Design review of the part built by this model. Coordinates are the model's own, in mm. Face numbers are marked on the shaded views. A direction names the side the tool comes from. Round coordinates to 2 decimals unless told otherwise and drop trailing zeros. Loops run counter-clockwise (first coordinate to the right, second up) from the corner with the lowest first, then second, coordinate; pieces in that order, holes last. Notation, with made-up numbers: (-10.5, 50) - (29.5, 50) arc R29 cw to (29.5, 84) - close; hole circle Ø9 at (-20, 31.5). An arc over 180 degrees is marked (long way). Return JSON: item names as keys, results as strings. Group by question number.
(1) We need section C-C, the plane z = -1.75. Write out the cut boundary in (x, y), and give its area (3 significant figures).
(2) Wall thickness on L1, parallel to X at y = 7.5, z = 10.15; L2, parallel to X at y = 10, z = 12; L3, parallel to Y at x = 78.5, z = 1: over which ranges is each line inside the solid? List them lowest first. Write a range as [from, to].
(3) For the marked faces 1 and 2, list the 3-axis set-ups (+Z, -Z, +X, -X, +Y, -Y) from which the entire face can be reached by the end or side of a thin tool; tool diameter is ignored.
(4) We need section B-B, the plane y = 22. Write out the cut boundary in (x, z).
(5) The part is to be moulded in two halves that separate along X. For the marked faces 3, 4, 5 and 6, say which applies: pulls with the +X half, pulls with the -X half, needs draft (parallel to the pull), parting line crosses it, or undercut.
(6) We need section D-D, the plane y = 51.5. Write out the cut boundary in (x, z), and give its area (3 significant figures).
(7) We need section A-A, the plane z = 2.25. Write out the cut boundary in (x, y).
(8) Clearance check with flat-ended pins moving along their axes: pin 1 (1 mm diameter, centred on x = 110.5, y = 28, fed in from -Z); pin 2 (5 mm diameter, centred on x = 87.5, y = 38.99, fed in from -Z); pin 3 (3 mm diameter, centred on x = 86.5, z = -2.5, fed in from -Y). State where each tip first meets the part, or that it passes through.
from build123d import *

# Parameters (mm, degrees)
SKETCH1_W           = 80
SKETCH1_H           = 18
SKETCH1_R           = 3
BOSS_EXTRUDE1_DEPTH = 20
SKETCH1_3_W         = 27.5
SKETCH1_3_H         = 18
SKETCH1_3_W_2       = 25
SKETCH1_3_R         = 3.5
BOSS_EXTRUDE2_DEPTH = 47
BOSS_EXTRUDE3_START = 47
SKETCH1_6_W         = 80
SKETCH1_6_H         = 18
BOSS_EXTRUDE3_DEPTH = 10
SKETCH2_R           = 5.5
SKETCH2_R_2         = 4.475
SKETCH2_R_3         = 3
BOSS_EXTRUDE4_DEPTH = 25
SKETCH2_6_R         = 10.5
SKETCH2_6_R_2       = 3
CUT_EXTRUDE5_DEPTH  = 161.097543738
SKETCH1_8_R         = 3
CUT_EXTRUDE6_DEPTH  = 57
CUT_EXTRUDE13_START = 27
SKETCH1_12_R        = 3
CUT_EXTRUDE13_DEPTH = 30
CUT_EXTRUDE14_START = -18
SKETCH2_7_W         = 9.3
SKETCH2_7_H         = 5
CUT_EXTRUDE14_DEPTH = 10


with BuildPart() as part:
    # Sketch1 → Boss-Extrude1 (new body)
    with BuildSketch(Plane(origin=(0, 0, 0), x_dir=(1, 0, 0), z_dir=(0, 1, 0))):
        with Locations((107.5033, -9)):
            Rectangle(SKETCH1_W, SKETCH1_H)
        with Locations(Location((135.5033, -10.15, 0), (0, 0, 270))):
            Circle(SKETCH1_R, mode=Mode.SUBTRACT)
        with Locations(Location((79.5033, -10.15, 0), (0, 0, 270))):
            Circle(SKETCH1_R, mode=Mode.SUBTRACT)
    extrude(amount=BOSS_EXTRUDE1_DEPTH)

    # Sketch1<3> → Boss-Extrude2 (add)
    # profile 1 of 11: a face of its own
    with BuildSketch(Plane(origin=(0, 0, 0), x_dir=(1, 0, 0), z_dir=(0, 1, 0))):
        with Locations((133.7533, -9)):
            Rectangle(SKETCH1_3_W, SKETCH1_3_H)
        Polygon((133.136163896, -6.05), (137.870436104, -6.05), (140.237572207, -10.15), (137.870436104, -14.25), (133.136163896, -14.25), (130.769027793, -10.15), align=None, mode=Mode.SUBTRACT)
    # profile 2 of 11: a face of its own
    with BuildSketch(Plane(origin=(0, 0, 0), x_dir=(1, 0, 0), z_dir=(0, 1, 0))):
        with Locations((81.2533, -9)):
            Rectangle(SKETCH1_3_W, SKETCH1_3_H)
        Polygon((81.88895579, -14.295097543), (77.154690915, -14.303429856), (74.780342483, -10.207602362), (77.140258926, -6.103442556), (81.874523801, -6.095110243), (84.248872233, -10.190937737), align=None, mode=Mode.SUBTRACT)
    # profile 3 of 11: a face of its own
    with BuildSketch(Plane(origin=(0, 0, 0), x_dir=(1, 0, 0), z_dir=(0, 1, 0))):
        with Locations((107.5033, -9)):
            Rectangle(SKETCH1_3_W_2, SKETCH1_3_H)
        with BuildLine():
            ThreePointArc((111.0033, -10.75), (107.5033, -14.25), (104.0033, -10.75))
            Line((104.0033, -10.75), (104.0033, -7.25))
            ThreePointArc((104.0033, -7.25), (107.5033, -3.75), (111.0033, -7.25))
            Line((111.0033, -7.25), (111.0033, -10.75))
        make_face(mode=Mode.SUBTRACT)
    # profile 4 of 11: a face of its own
    with BuildSketch(Plane(origin=(0, 0, 0), x_dir=(1, 0, 0), z_dir=(0, 1, 0))):
        with Locations((107.5033, -10.75)):
            Circle(SKETCH1_3_R)
    # profile 5 of 11: a face of its own
    with BuildSketch(Plane(origin=(0, 0, 0), x_dir=(1, 0, 0), z_dir=(0, 1, 0))):
        with Locations((107.5033, -7.25)):
            Circle(SKETCH1_3_R)
    # profile 6 of 11: a face of its own
    with BuildSketch(Plane(origin=(0, 0, 0), x_dir=(1, 0, 0), z_dir=(0, 1, 0))):
        with Locations((107.5033, -7.25)):
            Circle(SKETCH1_3_R)
    # profile 7 of 11: a face of its own
    with BuildSketch(Plane(origin=(0, 0, 0), x_dir=(1, 0, 0), z_dir=(0, 1, 0))):
        with Locations((107.5033, -10.75)):
            Circle(SKETCH1_3_R)
    # profile 8 of 11: a face of its own
    with BuildSketch(Plane(origin=(0, 0, 0), x_dir=(1, 0, 0), z_dir=(0, 1, 0))):
        with BuildLine():
            Line((104.0033, -7.25), (104.0033, -10.75))
            ThreePointArc((104.0033, -10.75), (104.122559608, -9.844133342), (104.472211087, -9))
            ThreePointArc((104.472211087, -9), (104.122559608, -8.155866658), (104.0033, -7.25))
        make_face()
    # profile 9 of 11: a face of its own
    with BuildSketch(Plane(origin=(0, 0, 0), x_dir=(1, 0, 0), z_dir=(0, 1, 0))):
        with BuildLine():
            ThreePointArc((110.534388913, -9), (110.884040392, -9.844133342), (111.0033, -10.75))
            Line((111.0033, -10.75), (111.0033, -7.25))
            ThreePointArc((111.0033, -7.25), (110.884040392, -8.155866658), (110.534388913, -9))
        make_face()
    # profile 10 of 11: a face of its own
    with BuildSketch(Plane(origin=(0, 0, 0), x_dir=(1, 0, 0), z_dir=(0, 1, 0))):
        with Locations((107.5033, -10.75)):
            Circle(SKETCH1_3_R)
    # profile 11 of 11: a face of its own
    with BuildSketch(Plane(origin=(0, 0, 0), x_dir=(1, 0, 0), z_dir=(0, 1, 0))):
        with Locations((107.5033, -7.25)):
            Circle(SKETCH1_3_R)
    extrude(amount=BOSS_EXTRUDE2_DEPTH)

    # Sketch1<6> → Boss-Extrude3 (add)
    with BuildSketch(Plane(origin=(0, 0, 0), x_dir=(1, 0, 0), z_dir=(0, 1, 0)).offset(BOSS_EXTRUDE3_START)):
        with Locations((107.5033, -9)):
            Rectangle(SKETCH1_6_W, SKETCH1_6_H)
        Polygon((133.136163896, -6.05), (137.870436104, -6.05), (140.237572207, -10.15), (137.870436104, -14.25), (133.136163896, -14.25), (130.769027793, -10.15), align=None, mode=Mode.SUBTRACT)
        with BuildLine():
            Line((104.0033, -10.75), (104.0033, -7.25))
            ThreePointArc((104.0033, -7.25), (107.5033, -3.75), (111.0033, -7.25))
            Line((111.0033, -7.25), (111.0033, -10.75))
            ThreePointArc((111.0033, -10.75), (107.5033, -14.25), (104.0033, -10.75))
        make_face(mode=Mode.SUBTRACT)
        Polygon((77.154690915, -14.303429856), (74.780342483, -10.207602362), (77.140258926, -6.103442556), (81.874523801, -6.095110243), (84.248872233, -10.190937737), (81.88895579, -14.295097543), align=None, mode=Mode.SUBTRACT)
    extrude(amount=BOSS_EXTRUDE3_DEPTH)

    # Sketch2 → Boss-Extrude4 (add)
    # profile 1 of 4: a face of its own
    with BuildSketch(Plane.XY.offset(18)):
        with Locations((87.5033, 38.99)):
            Circle(SKETCH2_R)
        with Locations((87.5033, 38.99)):
            Circle(SKETCH2_R_2, mode=Mode.SUBTRACT)
    # profile 2 of 4: a face of its own
    with BuildSketch(Plane.XY.offset(18)):
        with Locations((87.5033, 38.99)):
            Circle(SKETCH2_R_2)
        with Locations((87.5033, 38.99)):
            Circle(SKETCH2_R_3, mode=Mode.SUBTRACT)
    # profile 3 of 4: a face of its own
    with BuildSketch(Plane.XY.offset(18)):
        with Locations((127.5033, 38.99)):
            Circle(SKETCH2_R)
        with Locations((127.5033, 38.99)):
            Circle(SKETCH2_R_2, mode=Mode.SUBTRACT)
    # profile 4 of 4: a face of its own
    with BuildSketch(Plane.XY.offset(18)):
        with Locations((127.5033, 38.99)):
            Circle(SKETCH2_R_2)
        with Locations((127.5033, 38.99)):
            Circle(SKETCH2_R_3, mode=Mode.SUBTRACT)
    extrude(amount=-BOSS_EXTRUDE4_DEPTH)

    # Sketch2<6> → Cut-Extrude5 (cut, through all)
    with BuildSketch(Plane.XY.offset(18)):
        with Locations((107.5033, 39.05)):
            Circle(SKETCH2_6_R)
        with Locations((87.5033, 38.99)):
            Circle(SKETCH2_6_R_2)
        with Locations((127.5033, 38.99)):
            Circle(SKETCH2_6_R_2)
    extrude(amount=-CUT_EXTRUDE5_DEPTH, mode=Mode.SUBTRACT)

    # Sketch1<8> → Cut-Extrude6 (cut)
    with BuildSketch(Plane(origin=(0, 0, 0), x_dir=(1, 0, 0), z_dir=(0, 1, 0))):
        with Locations(Location((135.5033, -10.15, 0), (0, 0, 270))):
            Circle(SKETCH1_8_R)
        with Locations(Location((79.5033, -10.15, 0), (0, 0, 270))):
            Circle(SKETCH1_8_R)
    extrude(amount=CUT_EXTRUDE6_DEPTH, mode=Mode.SUBTRACT)

    # Sketch1<12> → Cut-Extrude13 (cut)
    # profile 1 of 2: a face of its own
    with BuildSketch(Plane(origin=(0, 0, 0), x_dir=(1, 0, 0), z_dir=(0, 1, 0)).offset(CUT_EXTRUDE13_START)):
        Polygon((137.870436104, -14.25), (140.237572207, -10.15), (137.870436104, -6.05), (133.136163896, -6.05), (130.769027793, -10.15), (133.136163896, -14.25), align=None)
        with Locations(Location((135.5033, -10.15, 0), (0, 0, 270))):
            Circle(SKETCH1_12_R, mode=Mode.SUBTRACT)
    # profile 2 of 2: a face of its own
    with BuildSketch(Plane(origin=(0, 0, 0), x_dir=(1, 0, 0), z_dir=(0, 1, 0)).offset(CUT_EXTRUDE13_START)):
        Polygon((77.140258926, -6.103442556), (81.874523801, -6.095110243), (84.248872233, -10.190937737), (81.88895579, -14.295097543), (77.154690915, -14.303429856), (74.780342483, -10.207602362), align=None)
        with Locations(Location((79.5033, -10.15, 0), (0, 0, 270))):
            Circle(SKETCH1_12_R, mode=Mode.SUBTRACT)
    extrude(amount=CUT_EXTRUDE13_DEPTH, mode=Mode.SUBTRACT)

    # Sketch2<7> → Cut-Extrude14 (cut)
    with BuildSketch(Plane.XY.offset(18).offset(CUT_EXTRUDE14_START)):
        with Locations((79.5033, 28.5)):
            Rectangle(SKETCH2_7_W, SKETCH2_7_H)
        with Locations((135.5033, 28.5)):
            Rectangle(SKETCH2_7_W, SKETCH2_7_H)
    extrude(amount=CUT_EXTRUDE14_DEPTH, mode=Mode.SUBTRACT)


solid = part.part
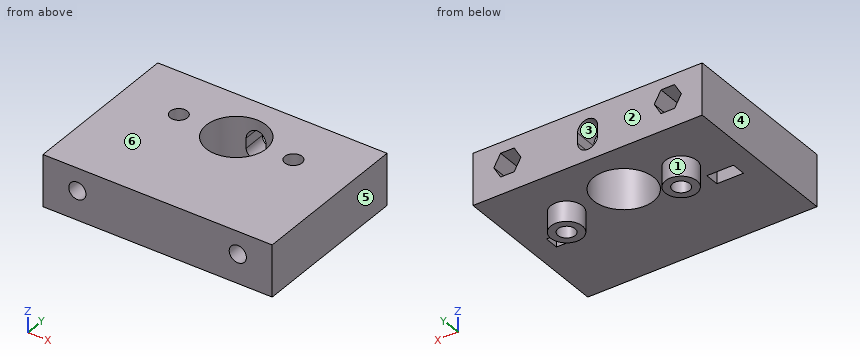
Solutions:
{
 "1": {"outline": "circle Ø11 at (87.5, 38.99); circle Ø11 at (127.5, 38.99); hole circle Ø6 at (87.5, 38.99); hole circle Ø6 at (127.5, 38.99)", "area": "134 mm^2"},
 "2": {"L1": "[67.5, 76.5], [82.5, 132.5], [138.5, 147.5]", "L2": "[67.5, 77.14], [81.86, 133.14], [137.86, 147.5]", "L3": "[0, 26], [31, 57]"},
 "3": {"face 1": "-Z", "face 2": "+Z, -Z, +X, -X, +Y"},
 "4": {"outline": "(67.5, 0) - (147.5, 0) - (147.5, 18) - (67.5, 18) - close; hole (74.78, 10.21) - (77.14, 6.1) - (81.87, 6.1) - (84.25, 10.19) - (81.89, 14.3) - (77.15, 14.3) - close; hole (130.77, 10.15) - (133.14, 6.05) - (137.87, 6.05) - (140.24, 10.15) - (137.87, 14.25) - (133.14, 14.25) - close"},
 "5": {"face 3": "undercut", "face 4": "pulls with the -X half", "face 5": "pulls with the +X half", "face 6": "needs draft"},
 "6": {"outline": "(67.5, 0) - (147.5, 0) - (147.5, 18) - (67.5, 18) - close; hole (74.78, 10.21) - (77.14, 6.1) - (81.87, 6.1) - (84.25, 10.19) - (81.89, 14.3) - (77.15, 14.3) - close; hole (104, 7.25) arc R3.5 ccw to (111, 7.25) - (111, 10.75) arc R3.5 ccw to (104, 10.75) - close; hole (130.77, 10.15) - (133.14, 6.05) - (137.87, 6.05) - (140.24, 10.15) - (137.87, 14.25) - (133.14, 14.25) - close", "area": "1,260 mm^2"},
 "7": {"outline": "(67.5, 0) - (147.5, 0) - (147.5, 57) - (67.5, 57) - close; hole (74.85, 26) - (84.15, 26) - (84.15, 31) - (74.85, 31) - close; hole circle Ø6 at (87.5, 38.99); hole circle Ø21 at (107.5, 39.05); hole circle Ø6 at (127.5, 38.99); hole (130.85, 26) - (140.15, 26) - (140.15, 31) - (130.85, 31) - close"},
 "8": {"pin 1": "z = 0", "pin 2": "through", "pin 3": "y = 33.49"}
}
